```python
from build123d import *

# Parameters (mm, degrees)
SKETCH_1_R          = 5.5
EXTRUDE_1_DEPTH     = 7
CUT_EXTRUDE_START   = -1
SKETCH_2_R          = 5.5
CUT_EXTRUDE_1_DEPTH = 1
EXTRUDE_2_DEPTH     = 1
SKETCH_5_W          = 4
SKETCH_5_H          = 4
CUT_EXTRUDE_2_DEPTH = 3
FILLET_3_R          = 1
FILLET_4_R          = 0.5


with BuildPart() as part:
    # Эскиз1 → Бобышка-Вытянуть1 (new body)
    with BuildSketch(Plane(origin=(0, 0, 0), x_dir=(1, 0, 0), z_dir=(0, 1, 0))):
        with Locations(Location((0, 0, 0), (0, 0, 270))):
            Circle(SKETCH_1_R)
    extrude(amount=EXTRUDE_1_DEPTH)

    # Эскиз6 → Повернуть3 (revolve)
    with BuildSketch(Plane.XY, mode=Mode.PRIVATE) as revolve_3_sk:
        with BuildLine():
            Line((-4.665230635, 2), (-7, 2))
            Line((-7, 2), (-7, 3))
            Line((-7, 3), (-7, 5.035898385))
            ThreePointArc((-7, 5.035898385), (-6.582112259, 6.271585962), (-5.5, 7))
            Line((-5.5, 7), (-4.665230635, 7))
            Line((-4.665230635, 7), (-4.665230635, 3))
            Line((-4.665230635, 3), (-4.665230635, 2))
        make_face()
    revolve(revolve_3_sk.sketch.rotate(Axis((0, -1000, 0), (0, 1, 0)), 180), axis=Axis((0, -1000, 0), (0, 1, 0)))

    # Эскиз2 → Вырез-Вытянуть1 (cut)
    with BuildSketch(Plane(origin=(0, 7, 0), x_dir=(1, 0, 0), z_dir=(0, 1, 0)).offset(CUT_EXTRUDE_START)):
        with Locations(Location((0, 0, 0), (0, 0, 180))):
            Circle(SKETCH_2_R)
    extrude(amount=CUT_EXTRUDE_1_DEPTH, mode=Mode.SUBTRACT)

    # Эскиз3 → Бобышка-Вытянуть2 (add)
    with BuildSketch(Plane(origin=(0, 6, 0), x_dir=(1, 0, 0), z_dir=(0, 1, 0))):
        Polygon((0, 4), (-4, 0), (-1.7, 0), (-1.7, -3.640107036), (1.7, -3.640107036), (1.7, 0), (4, 0), align=None)
    extrude(amount=EXTRUDE_2_DEPTH)

    # Эскиз5 → Вырез-Вытянуть2 (cut)
    with BuildSketch(Plane.XZ):
        Rectangle(SKETCH_5_W, SKETCH_5_H)
    extrude(amount=-CUT_EXTRUDE_2_DEPTH, mode=Mode.SUBTRACT)

    # Скругление3
    fillet_3_edges = [part.edges().sort_by_distance(p)[0] for p in [
        (5.5, 6, 0),
    ]]
    fillet(fillet_3_edges, radius=FILLET_3_R - 0.0001)  # a hair under: the kernel refuses the full size

    # Скругление4
    fillet_4_edges = [part.edges().sort_by_distance(p)[0] for p in [
        (2, 7, -2),
        (-2, 7, -2),
        (-2.85, 7, 0),
        (-1.7, 7, 1.820053518),
        (0, 7, 3.640107036),
        (1.7, 7, 1.820053518),
        (2.85, 7, 0),
    ]]
    fillet(fillet_4_edges, radius=FILLET_4_R)


solid = part.part
```
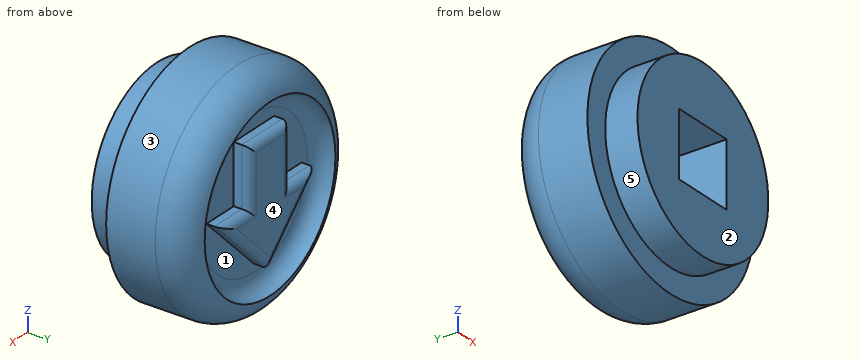
Source: CAD feature listing. Evaluate the final solid. Frame: model axes, mm. Face numbers are marked on the shaded views. A direction names the side the tool comes from. Give positions to 0.01 mm unless a question says otherwise; leave off trailing zeros. Order: outer loops, then holes, each group sorted by start corner. A loop starts at its lowest first (then second) coordinate and runs counter-clockwise, first axis right, second up.
(1) Access query for the marked faces 4 and 5. Directions: +Z, -Z, +X, -X, +Y, -Y. A direction counts if a zero-diameter tool reaches every point of the face in a straight line with its end or side. Return the directions, or none.
(2) Section query B-B (y = 1). Return the cut outline in (x, z), plus the area to 3 significant figures.
(3) Contact query for flat-ended pins moving along their axis: P1, Ø2.5, axis at x = -2, z = 1, coming from the +Y side; P2, Ø3, axis at x = 2, y = 3, coming from the -Z side; P3, Ø0.6, axis at y = 6.5, z = 2.5, coming from the +X side; P4, Ø0.6, axis at x = -2.5, y = 6.5, coming from the +Z side. Output: stop coordinate, or through.
(4) Section query A-A (y = 6.25). Return the cut outline in (x, z), plus the area to 3 significant figures.
(5) Pull-direction query (Z, two-part tool) for the marked faces 1, 2 and 3; classes: +Z half, -Z half, draft (parallel to the pull), parting line (faces both ways), or undercut.
(6) Section query C-C (y = 4.5). Return the cut outline in (x, z), plus the area to 3 significant figures.
(7) Material intervals for line 1 along Z through (x, y) = (1, 6.25); line 2 along Z through (x, y) = (-2, 6.25); line 3 along Y through (x, z) = (-1.75, 4.25), sorted ascending.
Outcome:
1. face 4: +Z, -Z, +X, -X, +Y
1. face 5: -Y
2. outline: circle Ø11 at (0, 0); hole (-2, -2) - (2, -2) - (2, 2) - (-2, 2) - close
2. area: 79.0 mm2
3. P1: stops at y = 7
3. P2: stops at z = -6.98
3. P3: stops at x = 6.17
3. P4: stops at z = 6.17
4. outline: circle Ø13.2 at (0, 0); (-4, 0) - (0, -4) - (4, 0) - (1.7, 0) - (1.7, 3.64) - (-1.7, 3.64) - (-1.7, 0) - close; hole circle Ø10.32 at (0, 0)
4. area: 81.5 mm2
5. face 1: undercut
5. face 2: draft
5. face 3: parting line
6. outline: circle Ø14 at (0, 0)
6. area: 154 mm2
7. line 1: z = -6.52 to -5.06, -3 to 3.64, 5.06 to 6.52
7. line 2: z = -6.29 to -4.76, -2 to 0, 4.76 to 6.29
7. line 3: y = 0 to 6
